Work out the finished part from the listing and answer in its coordinate system (mm). Face numbers are marked on the shaded views. A direction names the side the tool comes from. Round coordinates to 2 decimals unless told otherwise and drop trailing zeros. Use CSV: the item, a comma, the result in double quotes.
from build123d import *
from build123d.topology import SkipClean

# Parameters (mm, degrees)
REVOLU_O2_ANGLE          = 180
ESBO_O4_R                = 10
RESSALTO_EXTRUS_O1_DEPTH = 35
RESSALTO_EXTRUS_O2_DEPTH = 20
ESBO_O8_R                = 3.5
CORTE_EXTRUS_O2_DEPTH    = 20
PADR_OCIRCULAR1_COUNT    = 6
ESBO_O6_R                = 2.5
CORTE_EXTRUS_O1_DEPTH    = 15
ESBO_O9_R                = 1.25
CORTE_EXTRUS_O3_DEPTH    = 6
ESBO_O10_W               = 2.2
ESBO_O10_H               = 116.4
CORTE_EXTRUS_O4_DEPTH    = 3.5
ESBO_O11_W               = 2
ESBO_O11_H               = 114.9
RESSALTO_EXTRUS_O5_DEPTH = 2
ESBO_O12_R               = 3.25
RESSALTO_EXTRUS_O6_DEPTH = 20
ESBO_O13_R               = 2.5
RESSALTO_EXTRUS_O7_DEPTH = 20
CORTE_EXTRUS_O5_DEPTH    = 180.26806743
CORTE_EXTRUS_O6_START    = 10
ESBO_O16_R               = 93
CORTE_EXTRUS_O6_DEPTH    = 10
ESBO_O17_R               = 92.967356783
ESBO_O17_R_2             = 90.967356783
CORTE_EXTRUS_O7_DEPTH    = 1.5
ESBO_O18_W               = 100
ESBO_O18_H               = 17.238697901
CORTE_EXTRUS_O8_DEPTH    = 15
RESSALTO_EXTRUS_O9_DEPTH = 15
ESBO_O22_R               = 1.65
CORTE_EXTRUS_O9_DEPTH    = 10


with BuildPart() as part:
    # Esboço3 → Revolução2 (revolve)
    with BuildSketch(Plane.XY):
        with BuildLine():
            Line((97.5, 79.8), (97.5, 11.304491341))
            Line((97.5, 11.304491341), (97.5, 0))
            Line((97.5, 0), (97.5, -40.2))
            Line((97.5, -40.2), (87.5, -40.2))
            Line((87.5, -40.2), (87.5, 0))
            Line((87.5, 0), (60.342408243, 0))
            Line((60.342408243, 0), (60.342408243, 2.95))
            Line((60.342408243, 2.95), (52, 2.95))
            Line((52, 2.95), (44, 10.95))
            Line((44, 10.95), (31, 10.95))
            Line((31, 10.95), (31, 13.7))
            Line((31, 13.7), (22.6, 13.7))
            Line((22.6, 13.7), (22.6, 17))
            Line((22.6, 17), (19.3, 17))
            Line((19.3, 17), (19.3, 17.7))
            Line((19.3, 17.7), (15.3, 17.7))
            Line((15.3, 17.7), (15.3, 21.05))
            Line((15.3, 21.05), (19.3, 21.05))
            Line((19.3, 21.05), (19.3, 21.2))
            Line((19.3, 21.2), (27.626549127, 25.96))
            Line((27.626549127, 25.96), (31.3, 25.96))
            Line((31.3, 25.96), (31.3, 43.96))
            Line((31.3, 43.96), (32.3, 44.96))
            Line((32.3, 44.96), (38.8, 44.96))
            Line((38.8, 44.96), (38.8, 26.9))
            Line((38.8, 26.9), (55.5, 10.2))
            Line((55.5, 10.2), (83.5, 10.2))
            ThreePointArc((83.5, 10.2), (86.328427125, 11.371572875), (87.5, 14.2))
            Line((87.5, 14.2), (87.5, 76.2))
            Line((87.5, 76.2), (93, 76.2))
            Line((93, 76.2), (93, 79.8))
            Line((93, 79.8), (97.5, 79.8))
        make_face()
    revolve(axis=Axis((0, -3.322055656, 0), (0, 1, 0)), revolution_arc=REVOLU_O2_ANGLE)

    # Esboço20 → Revolução3 (revolve)
    with SkipClean():  # the faces are left unmerged after this step: merging them gives an invalid solid
        with BuildSketch(Plane.XY, mode=Mode.PRIVATE) as revolu_o3_sk:
            Polygon((60.342408243, 2.95), (60.342408243, 10.2), (55.5, 10.2), (38.8, 26.9), (38.8, 44.96), (32.3, 44.96), (31.3, 43.96), (31.3, 25.96), (27.626549127, 25.96), (19.3, 21.2), (19.3, 21.05), (15.3, 21.05), (15.3, 17.7), (19.3, 17.7), (19.3, 17), (22.6, 17), (22.6, 13.7), (31, 13.7), (31, 10.95), (44, 10.95), (52, 2.95), align=None)
        revolve(revolu_o3_sk.sketch.rotate(Axis((0, -3.322055656, 0), (0, 1, 0)), 90), axis=Axis((0, -3.322055656, 0), (0, 1, 0)))
    add(part.part.scale(1), mode=Mode.REPLACE)  # the faces are merged on a copy

    # Esboço4 → Ressalto-extrusão1 (add)
    with SkipClean():  # the faces are left unmerged after this step: merging them gives an invalid solid
        with BuildSketch(Plane(origin=(0, 79.8, 0), x_dir=(1, 0, 0), z_dir=(0, 1, 0))):
            with Locations((70.71, 70.71)):
                Circle(ESBO_O4_R)
            with Locations((-70.71, 70.71)):
                Circle(ESBO_O4_R)
        extrude(amount=-RESSALTO_EXTRUS_O1_DEPTH)

    # Esboço5 → Ressalto-extrusão2 (add)
    with SkipClean():  # the faces are left unmerged after this step: merging them gives an invalid solid
        with BuildSketch(Plane.XZ.offset(40.2)):
            with BuildLine():
                Line((10, -105), (10, -96.985823706))
                Line((10, -96.985823706), (-10, -96.985823706))
                Line((-10, -96.985823706), (-10, -105))
                ThreePointArc((-10, -105), (0, -115), (10, -105))
            make_face()
        ressalto_extrus_o2 = extrude(amount=-RESSALTO_EXTRUS_O2_DEPTH)

    # Esboço8 → Corte-extrusão2 (cut)
    with SkipClean():  # the faces are left unmerged after this step: merging them gives an invalid solid
        with BuildSketch(Plane.XZ.offset(40.2)):
            with Locations(Location((0, -105, 0), (0, 0, 270))):
                Circle(ESBO_O8_R)
        corte_extrus_o2 = extrude(amount=-CORTE_EXTRUS_O2_DEPTH, mode=Mode.SUBTRACT)

    # PadrãoCircular1: Ressalto-extrusão2, Corte-extrusão2 ×6 about axis, 3 skipped
    with SkipClean():  # the faces are left unmerged after this step: merging them gives an invalid solid
        padr_ocircular1_axis = Axis((0, 0, 0), (0, 1, 0))
        add([ressalto_extrus_o2.rotate(padr_ocircular1_axis, i * 360 / PADR_OCIRCULAR1_COUNT) for i in range(1, PADR_OCIRCULAR1_COUNT) if i not in (2, 3, 4)])
        add([corte_extrus_o2.rotate(padr_ocircular1_axis, i * 360 / PADR_OCIRCULAR1_COUNT) for i in range(1, PADR_OCIRCULAR1_COUNT) if i not in (2, 3, 4)], mode=Mode.SUBTRACT)

    # Esboço6 → Corte-extrusão1 (cut)
    with SkipClean():  # the faces are left unmerged after this step: merging them gives an invalid solid
        with BuildSketch(Plane(origin=(0, 79.8, 0), x_dir=(1, 0, 0), z_dir=(0, 1, 0))):
            with Locations(Location((70.71, 70.71, 0), (0, 0, 270))):
                Circle(ESBO_O6_R)
            with Locations(Location((-70.71, 70.71, 0), (0, 0, 270))):
                Circle(ESBO_O6_R)
        extrude(amount=-CORTE_EXTRUS_O1_DEPTH, mode=Mode.SUBTRACT)

    # Esboço9 → Corte-extrusão3 (cut)
    with SkipClean():  # the faces are left unmerged after this step: merging them gives an invalid solid
        with BuildSketch(Plane.XZ.offset(-13.7)):
            with Locations(Location((18.738329701, -18.738329701, 0), (0, 0, 270))):
                Circle(ESBO_O9_R)
            with Locations(Location((-18.738329701, -18.738329701, 0), (0, 0, 270))):
                Circle(ESBO_O9_R)
            with Locations(Location((-18.738329701, 18.738329701, 0), (0, 0, 270))):
                Circle(ESBO_O9_R)
            with Locations(Location((18.738329701, 18.738329701, 0), (0, 0, 270))):
                Circle(ESBO_O9_R)
        extrude(amount=-CORTE_EXTRUS_O3_DEPTH, mode=Mode.SUBTRACT)

    # Esboço10 → Corte-extrusão4 (cut)
    with SkipClean():  # the faces are left unmerged after this step: merging them gives an invalid solid
        with BuildSketch(Plane.XY):
            with Locations((92, 18)):
                Rectangle(ESBO_O10_W, ESBO_O10_H)
        extrude(amount=-CORTE_EXTRUS_O4_DEPTH, mode=Mode.SUBTRACT)

    # Esboço11 → Ressalto-extrusão5 (add)
    with SkipClean():  # the faces are left unmerged after this step: merging them gives an invalid solid
        with BuildSketch(Plane.XY):
            with Locations((-92, 18.75)):
                Rectangle(ESBO_O11_W, ESBO_O11_H)
        extrude(amount=RESSALTO_EXTRUS_O5_DEPTH)

    # Esboço12 → Ressalto-extrusão6 (add)
    with BuildSketch(Plane.XY):
        with BuildLine():
            Line((-102, 29.8), (-87.5, 29.8))
            Line((-87.5, 29.8), (-87.5, 9.8))
            Line((-87.5, 9.8), (-102, 9.8))
            ThreePointArc((-102, 9.8), (-112, 19.8), (-102, 29.8))
        make_face()
        with Locations((-102, 19.8)):
            Circle(ESBO_O12_R, mode=Mode.SUBTRACT)
    extrude(amount=-RESSALTO_EXTRUS_O6_DEPTH)

    # Esboço13 → Ressalto-extrusão7 (add)
    with BuildSketch(Plane.XY):
        with BuildLine():
            Line((102, 29.8), (93.1, 29.8))
            Line((93.1, 29.8), (93.1, 9.8))
            Line((93.1, 9.8), (102, 9.8))
            ThreePointArc((102, 9.8), (112, 19.8), (102, 29.8))
        make_face()
        with Locations((102, 19.8)):
            Circle(ESBO_O13_R, mode=Mode.SUBTRACT)
    extrude(amount=-RESSALTO_EXTRUS_O7_DEPTH)

    # Esboço14 → Corte-extrusão5 (cut, through all)
    with SkipClean():  # the faces are left unmerged after this step: merging them gives an invalid solid
        with BuildSketch(Plane(origin=(0, 0, 0), x_dir=(-1, 0, 0), z_dir=(0, -1, 0))):
            with BuildLine():
                ThreePointArc((34.350508428, 67.496062714), (0, 70), (-34.350508428, 67.496062714))
                ThreePointArc((-34.350508428, 67.496062714), (-47.016691783, 50.479370931), (-30, 37.813187576))
                ThreePointArc((-30, 37.813187576), (0, 40), (30, 37.813187576))
                ThreePointArc((30, 37.813187576), (47.016691783, 50.479370931), (34.350508428, 67.496062714))
            make_face()
        extrude(amount=-CORTE_EXTRUS_O5_DEPTH, mode=Mode.SUBTRACT)

    # Esboço16 → Corte-extrusão6 (cut)
    with SkipClean():  # the faces are left unmerged after this step: merging them gives an invalid solid
        with BuildSketch(Plane(origin=(0, 76.2, 0), x_dir=(1, 0, 0), z_dir=(0, 1, 0)).offset(CORTE_EXTRUS_O6_START)):
            Circle(ESBO_O16_R)
        extrude(amount=-CORTE_EXTRUS_O6_DEPTH, mode=Mode.SUBTRACT)

    # Esboço17 → Corte-extrusão7 (cut)
    with SkipClean():  # the faces are left unmerged after this step: merging them gives an invalid solid
        with BuildSketch(Plane.XZ.offset(40.2)):
            Circle(ESBO_O17_R)
            Circle(ESBO_O17_R_2, mode=Mode.SUBTRACT)
        extrude(amount=-CORTE_EXTRUS_O7_DEPTH, mode=Mode.SUBTRACT)

    # Esboço18 → Corte-extrusão8 (cut, symmetric)
    with SkipClean():  # the faces are left unmerged after this step: merging them gives an invalid solid
        with BuildSketch(Plane(origin=(0, -20.1, 0), x_dir=(-1, 0, 0), z_dir=(0, -1, 0))):
            with Locations((0, 72.662310295)):
                Rectangle(ESBO_O18_W, ESBO_O18_H)
        extrude(amount=CORTE_EXTRUS_O8_DEPTH, both=True, mode=Mode.SUBTRACT)

    # Esboço19 → Ressalto-extrusão9 (add, symmetric)
    with SkipClean():  # the faces are left unmerged after this step: merging them gives an invalid solid
        with BuildSketch(Plane(origin=(0, -20.1, 0), x_dir=(-1, 0, 0), z_dir=(0, -1, 0))):
            with BuildLine():
                Line((32.396633626, 81.281659245), (-32.396633626, 81.281659245))
                ThreePointArc((-32.396633626, 81.281659245), (0, 87.5), (32.396633626, 81.281659245))
            make_face()
        extrude(amount=RESSALTO_EXTRUS_O9_DEPTH, both=True)

    # Esboço22 → Corte-extrusão9 (cut)
    with SkipClean():  # the faces are left unmerged after this step: merging them gives an invalid solid
        with BuildSketch(Plane.XY.offset(-81.281659245)):
            with Locations((-15.9, -24.1)):
                Circle(ESBO_O22_R)
            with Locations((15.9, -24.1)):
                Circle(ESBO_O22_R)
        extrude(amount=-CORTE_EXTRUS_O9_DEPTH, mode=Mode.SUBTRACT)


solid = part.part
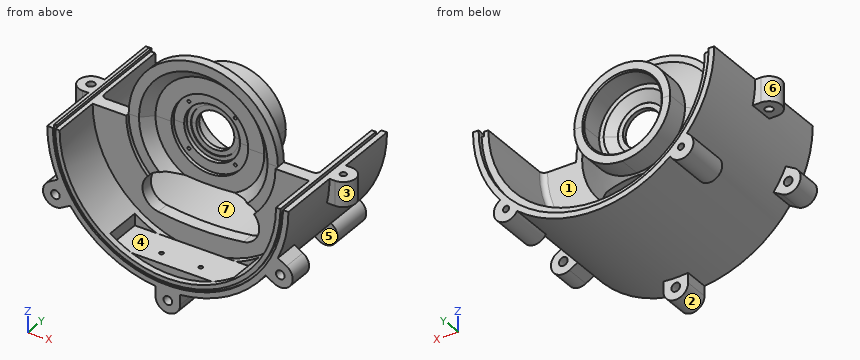
(1) Each of these flat-tipped pins is pushed along its axis until it touches: pin 1 (2 mm diameter, centred on x = -18.5, z = 18.5, fed in from -Y); pin 2 (7.5 mm diameter, centred on x = -42.5, z = -75, fed in from +Y); pin 3 (2 mm diameter, centred on x = -69, y = 61.5, fed in from +Z); pin 4 (6 mm diameter, centred on x = -21, z = -88.5, fed in from +Y). Where does it stop, or does it pass through?
Findings below:
pin 1,"stops at y = 13.7"
pin 2,"stops at y = 76.2"
pin 3,"stops at z = -52.5"
pin 4,"stops at y = 79.8"
(2) The mould has two halves that part along Y. Classify the marked faces 1, 2, 3 and 4: released by +Y, released by -Y, zero draft, split by the parting line, or undercut.
Findings below:
face 1,"released by +Y"
face 2,"zero draft"
face 3,"split by the parting line"
face 4,"undercut"
(3) Find the intervals of material crossed by L1, parallel to Y at x = -102, z = -11.75; L2, parallel to X at y = 76.75, z = -70.71; L3, parallel to X at y = -32, z = -52.5, in increasing order. Write a range as from..to.
Findings below:
L1,"y = 9.8..16.55, 23.05..29.8"
L2,"x = -80.71..-73.21, -68.21..-60.41, 60.41..68.21, 73.21..80.71"
L3,"x = -100.93..-94.43, -87.43..-70, 70..87.43, 94.43..100.93"
(4) For the marked faces 5, 6 and 7, determine the directions among +Z, -Z, +X, -X, +Y, -Y from which every point of the face is accessible in a straight line to the end or side of a thin tool.
Findings below:
face 5,"-Z, +X, -Y"
face 6,"+Z, -Z, -X"
face 7,"+Y"
